```python
from build123d import *

# Parameters (mm, degrees)
F0_W     = 40
F0_H     = 25
F0_R     = 8
F1_DEPTH = 8
F3_DEPTH = 8


# Not quite as in the source:
# - a feature of the source that left no trace in its solid (it failed there, or was rolled back) is left out


with BuildPart() as f1:
    # F0 (on Top) → F1 (new body)
    with BuildSketch(Plane.XY):
        Rectangle(F0_W, F0_H)
        with Locations((7, 0)):
            Circle(F0_R, mode=Mode.SUBTRACT)
    extrude(amount=F1_DEPTH)

    # F2 (on face) → F3 (cut, through all)
    with BuildSketch(Plane.XY.offset(8)):
        with BuildLine():
            Line((-1, 12.5), (-1, 0))
            ThreePointArc((-1, 0), (7, 8), (15, 0))
            Line((15, 0), (15, 12.5))
            Line((15, 12.5), (-1, 12.5))
        make_face()
    extrude(amount=-F3_DEPTH, mode=Mode.SUBTRACT)


solid = f1.part
```
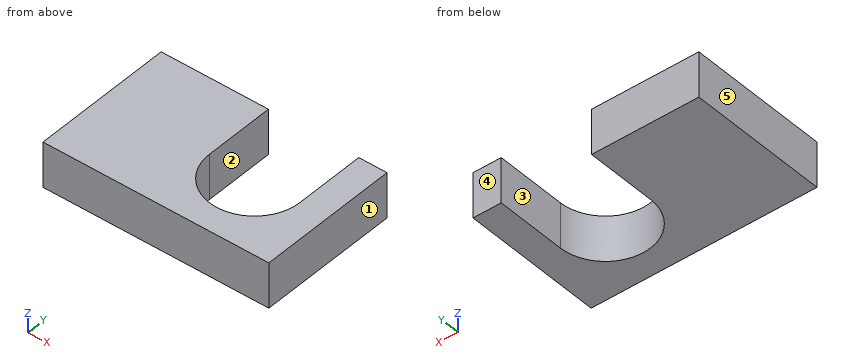
The listing builds one solid part. Answer for the finished solid, in the listing's coordinates (mm). Face numbers are marked on the shaded views. A direction names the side the tool comes from. Round coordinates to 2 decimals unless told otherwise and drop trailing zeros. Loops run counter-clockwise (first coordinate to the right, second up) from the corner with the lowest first, then second, coordinate; pieces in that order, holes last.
1) A cutting plane is placed at B-B on z = 0.5. Determine the outline of the cut face in (x, y), plus the area to 3 significant figures.
Outcome:
outline: (-20, -12.5) - (20, -12.5) - (20, 12.5) - (15, 12.5) - (15, 0) arc R8 cw to (-1, 0) - (-1, 12.5) - (-20, 12.5) - close
area: 699 mm2
2) A cutting plane is placed at A-A on y = 9. Determine the outline of the cut face in (x, z).
Outcome:
outline: (-20, 0) - (-1, 0) - (-1, 8) - (-20, 8) - close; (15, 0) - (20, 0) - (20, 8) - (15, 8) - close
3) A cutting plane is placed at C-C on x = 7. Determine the outline of the cut face in (y, z), plus the area to 3 significant figures.
Outcome:
outline: (-12.5, 0) - (-8, 0) - (-8, 8) - (-12.5, 8) - close
area: 36.0 mm2
4) Consider line 1 (X direction, y = 4.75, z = 2); line 2 (X direction, y = -6.5, z = 1); line 3 (Y direction, x = 9, z = 1). Determine where each line is inside the solid, lowest interval first.
Outcome:
line 1: x = -20 to -1, 15 to 20
line 2: x = -20 to 2.34, 11.66 to 20
line 3: y = -12.5 to -7.75
5) For a pull along X with two mould halves and no side action, classify the marked faces 3, 4 and 5 as released by +X, released by -X, zero draft, split by the parting line, or undercut.
Outcome:
face 3: undercut
face 4: zero draft
face 5: released by -X
6) A cutting plane is placed at D-D on x = 14.5. Determine the outline of the cut face in (y, z), plus the area to 3 significant figures.
Outcome:
outline: (-12.5, 0) - (-2.78, 0) - (-2.78, 8) - (-12.5, 8) - close
area: 77.7 mm2
7) For the marked faces 1 and 2, determine the directions among +Z, -Z, +X, -X, +Y, -Y from which every point of the face is accessible in a straight line to the end or side of a thin tool.
Outcome:
face 1: +Z, -Z, +X, +Y, -Y
face 2: +Z, -Z, +Y
8) Given P1, Ø8, axis at x = -11, y = 6, coming from the -Z side, flat-ended and moving along its own axis, determine where the tip first touches the part or whether it passes through.
Outcome:
P1: stops at z = 0
